Input: part model. Units: mm. Frame: model coordinates. A direction names the side the tool comes from. Coordinates: 2 decimals unless noted, no trailing zeros. Order: outer loops, then holes, each group sorted by start corner. A loop starts at its lowest first (then second) coordinate and runs counter-clockwise, first axis right, second up. Notation, with made-up numbers: (-18, -10) - (20, -10) arc R24 ccw to (20, 17) - close; hole circle Ø5 at (74, 79.25). An arc over 180 degrees is marked (long way). Use a Markdown table: item, result. Add a question column.
from build123d import *

# Parameters (mm, degrees)
BODY_DEPTH                    = 6
SKETCH2_W                     = 10.280011329
SKETCH2_H                     = 42.3
SKETCH2_W_2                   = 2
WINGS_DEPTH                   = 130
SKETCH3_R                     = 1.6
MOUNTING_BORE_DEPTH           = 152.726728034
CUT_EXCESS_MATERIAL_DEPTH     = 175.702604445
CUT_BATTERY_MOUNT_REACH       = 153.727
SKETCH6_R                     = 1.6
SKETCH8_W                     = 6.8
SKETCH8_H                     = 2.8
CAPTURE_NUT_1_DEPTH           = 7.3
CIRPATTERN1_COUNT             = 2
SKETCH10_W                    = 6.8
SKETCH10_H                    = 2.8
CAPTURE_NUT_2_DEPTH           = 7.3
CIRPATTERN2_COUNT             = 2
CUT_CENTER_HOLE_REACH         = 153.727
SKETCH11_R                    = 30
CUT_HARNESS_MOUNT_REACH       = 153.727
SKETCH12_R                    = 2.5
CAPTIVE_NUT_WALL_1_DEPTH      = 2.8
CAPTIVE_NUT_WALL_2_REACH      = 147.131
CAPTIVE_NUT_WALL_3_REACH      = 147.131
CAPTIVE_NUT_WALL_4_REACH      = 147.131
MIDDLE_DECK_HOLES_REACH       = 161.285
SKETCH20_R                    = 1.6
MIDDLE_DECK_CAPTIVE_NUT_DEPTH = 2.5
WING_EXTRA_WIDTH_1_DEPTH      = 3
WING_EXTRA_WIDTH_2_DEPTH      = 3


with BuildPart() as part:
    # Sketch1 → body (new body)
    with BuildSketch(Plane(origin=(0, 0, 0), x_dir=(1, 0, 0), z_dir=(0, 1, 0))):
        with BuildLine():
            ThreePointArc((-39.719988671, -21.15), (-45, 0), (-39.719988671, 21.15))
            Line((-39.719988671, 21.15), (-50, 21.15))
            Line((-50, 21.15), (-50, -21.15))
            Line((-50, -21.15), (-39.719988671, -21.15))
        make_face()
        with BuildLine():
            Line((-16, -21.15), (-16, 21.15))
            Line((-16, 21.15), (-39.719988671, 21.15))
            ThreePointArc((-39.719988671, 21.15), (-45, 0), (-39.719988671, -21.15))
            Line((-39.719988671, -21.15), (-16, -21.15))
        make_face()
        with BuildLine():
            Line((-39.719988671, 21.15), (-16, 21.15))
            Line((-16, 21.15), (-16, -21.15))
            Line((-16, -21.15), (-39.719988671, -21.15))
            ThreePointArc((-39.719988671, -21.15), (0, -45), (39.719988671, -21.15))
            Line((39.719988671, -21.15), (16, -21.15))
            Line((16, -21.15), (16, 21.15))
            Line((16, 21.15), (39.719988671, 21.15))
            ThreePointArc((39.719988671, 21.15), (0, 45), (-39.719988671, 21.15))
        make_face()
        with BuildLine():
            ThreePointArc((45, 0), (43.66004747, 10.899552968), (39.719988671, 21.15))
            Line((39.719988671, 21.15), (16, 21.15))
            Line((16, 21.15), (16, -21.15))
            Line((16, -21.15), (39.719988671, -21.15))
            ThreePointArc((39.719988671, -21.15), (43.66004747, -10.899552968), (45, 0))
        make_face()
        with BuildLine():
            Line((50, 21.15), (39.719988671, 21.15))
            ThreePointArc((39.719988671, 21.15), (43.66004747, 10.899552968), (45, 0))
            ThreePointArc((45, 0), (43.66004747, -10.899552968), (39.719988671, -21.15))
            Line((39.719988671, -21.15), (50, -21.15))
            Line((50, -21.15), (50, 21.15))
        make_face()
    extrude(amount=BODY_DEPTH)

    # Sketch2 → wings (add)
    with BuildSketch(Plane(origin=(0, 6, 0), x_dir=(1, 0, 0), z_dir=(0, 1, 0))):
        with Locations((44.859994336, 0)):
            Rectangle(SKETCH2_W, SKETCH2_H)
        with Locations((-44.859994336, 0)):
            Rectangle(SKETCH2_W, SKETCH2_H)
        with Locations((-38.719988671, 0)):
            Rectangle(SKETCH2_W_2, SKETCH2_H)
        with Locations((38.719988671, 0)):
            Rectangle(SKETCH2_W_2, SKETCH2_H)
    extrude(amount=WINGS_DEPTH)

    # Sketch3 → mounting-bore (cut, through all)
    with BuildSketch(Plane(origin=(0, 136, 0), x_dir=(1, 0, 0), z_dir=(0, 1, 0))):
        with Locations(Location((43, -17.5, 0), (0, 0, 270))):
            Circle(SKETCH3_R)
        with Locations(Location((-43, -17.5, 0), (0, 0, 270))):
            Circle(SKETCH3_R)
        with Locations(Location((-43, 17.5, 0), (0, 0, 270))):
            Circle(SKETCH3_R)
        with Locations(Location((43, 17.5, 0), (0, 0, 270))):
            Circle(SKETCH3_R)
    extrude(amount=-MOUNTING_BORE_DEPTH, mode=Mode.SUBTRACT)

    # Sketch5 → cut-excess-material (cut, through all)
    with BuildSketch(Plane(origin=(50, 0, 0), x_dir=(0, 0, -1), z_dir=(1, 0, 0))):
        Polygon((0, 6), (9, 6), (9, 136), (-9, 136), (-9, 6), align=None)
    extrude(amount=-CUT_EXCESS_MATERIAL_DEPTH, mode=Mode.SUBTRACT)

    # Sketch6 → cut-battery-mount (cut, up to next)
    with BuildSketch(Plane.XZ, mode=Mode.PRIVATE) as cut_battery_mount_sk1:
        with Locations(Location((-44, 0, 0), (0, 0, 270))):
            Circle(SKETCH6_R)
    cut_battery_mount_tool1 = extrude(cut_battery_mount_sk1.sketch, amount=-CUT_BATTERY_MOUNT_REACH, mode=Mode.PRIVATE) & part.part
    # Sketch6 → cut-battery-mount (cut, up to next)
    with BuildSketch(Plane.XZ, mode=Mode.PRIVATE) as cut_battery_mount_sk2:
        with Locations(Location((44, 0, 0), (0, 0, 270))):
            Circle(SKETCH6_R)
    cut_battery_mount_tool2 = extrude(cut_battery_mount_sk2.sketch, amount=-CUT_BATTERY_MOUNT_REACH, mode=Mode.PRIVATE) & part.part
    add(cut_battery_mount_tool1.solids().sort_by_distance((-44, 0, 0))[0], mode=Mode.SUBTRACT)
    add(cut_battery_mount_tool2.solids().sort_by_distance((44, 0, 0))[0], mode=Mode.SUBTRACT)

    # Sketch8 → capture-nut-1 (cut)
    with BuildSketch(Plane.XY.offset(21.15)):
        with Locations((42.999988671, 130)):
            Rectangle(SKETCH8_W, SKETCH8_H)
    capture_nut_1 = extrude(amount=-CAPTURE_NUT_1_DEPTH, mode=Mode.SUBTRACT)

    # CirPattern1: capture-nut-1 ×2 about axis
    cirpattern1_axis = Axis((0, 0, 0), (0, 1, 0))
    for i in range(1, CIRPATTERN1_COUNT):
        add(capture_nut_1.rotate(cirpattern1_axis, i * 360 / CIRPATTERN1_COUNT), mode=Mode.SUBTRACT)

    # Sketch10 → capture-nut-2 (cut)
    with BuildSketch(Plane(origin=(0, 0, -21.15), x_dir=(-1, 0, 0), z_dir=(0, 0, -1))):
        with Locations((-42.999988671, 130)):
            Rectangle(SKETCH10_W, SKETCH10_H)
    capture_nut_2 = extrude(amount=-CAPTURE_NUT_2_DEPTH, mode=Mode.SUBTRACT)

    # CirPattern2: capture-nut-2 ×2 about axis
    cirpattern2_axis = Axis((0, 0, 0), (0, 1, 0))
    for i in range(1, CIRPATTERN2_COUNT):
        add(capture_nut_2.rotate(cirpattern2_axis, i * 360 / CIRPATTERN2_COUNT), mode=Mode.SUBTRACT)

    # Sketch11 → cut-center-hole (cut, up to next)
    with BuildSketch(Plane.XZ, mode=Mode.PRIVATE) as cut_center_hole_sk1:
        with Locations(Location((0, 0, 0), (0, 0, 270))):
            Circle(SKETCH11_R)
    cut_center_hole_tool1 = extrude(cut_center_hole_sk1.sketch, amount=-CUT_CENTER_HOLE_REACH, mode=Mode.PRIVATE) & part.part
    add(cut_center_hole_tool1.solids().sort_by_distance((0, 0, 0))[0], mode=Mode.SUBTRACT)

    # Sketch12 → cut-harness-mount (cut, up to next)
    with BuildSketch(Plane.XZ, mode=Mode.PRIVATE) as cut_harness_mount_sk1:
        with Locations(Location((0, -40, 0), (0, 0, 270))):
            Circle(SKETCH12_R)
    cut_harness_mount_tool1 = extrude(cut_harness_mount_sk1.sketch, amount=-CUT_HARNESS_MOUNT_REACH, mode=Mode.PRIVATE) & part.part
    # Sketch12 → cut-harness-mount (cut, up to next)
    with BuildSketch(Plane.XZ, mode=Mode.PRIVATE) as cut_harness_mount_sk2:
        with Locations(Location((0, 40, 0), (0, 0, 270))):
            Circle(SKETCH12_R)
    cut_harness_mount_tool2 = extrude(cut_harness_mount_sk2.sketch, amount=-CUT_HARNESS_MOUNT_REACH, mode=Mode.PRIVATE) & part.part
    add(cut_harness_mount_tool1.solids().sort_by_distance((0, 0, -40))[0], mode=Mode.SUBTRACT)
    add(cut_harness_mount_tool2.solids().sort_by_distance((0, 0, 40))[0], mode=Mode.SUBTRACT)

    # Sketch13 → captive-nut-wall-1 (add)
    with BuildSketch(Plane(origin=(0, 128.6, 0), x_dir=(1, 0, 0), z_dir=(0, 1, 0))):
        Polygon((46.399988671, 13.85), (46.399988671, 17.5), (44.699994335, 14.555523439), (41.300005665, 14.555523439), (39.600011329, 17.5), (39.599988671, 13.85), align=None)
    extrude(amount=CAPTIVE_NUT_WALL_1_DEPTH)

    # Sketch14 → captive-nut-wall-2 (add, up to next)
    with BuildSketch(Plane(origin=(0, 128.6, 0), x_dir=(1, 0, 0), z_dir=(0, 1, 0)), mode=Mode.PRIVATE) as captive_nut_wall_2_sk1:
        Polygon((-39.599988671, 13.85), (-39.599988671, 17.5), (-41.299994335, 14.555503816), (-44.700005665, 14.555503816), (-46.400011329, 17.5), (-46.400011329, 13.85), align=None)
    captive_nut_wall_2_tool1 = extrude(captive_nut_wall_2_sk1.sketch, amount=CAPTIVE_NUT_WALL_2_REACH, mode=Mode.PRIVATE) - part.part
    add(captive_nut_wall_2_tool1.solids().sort_by_distance((-39.677166, 128.6, -15.675))[0])

    # Sketch16 → captive-nut-wall-3 (add, up to next)
    with BuildSketch(Plane(origin=(0, 128.6, 0), x_dir=(1, 0, 0), z_dir=(0, 1, 0)), mode=Mode.PRIVATE) as captive_nut_wall_3_sk1:
        Polygon((-46.399988671, -13.85), (-46.399988671, -17.5), (-44.699994335, -14.555523439), (-41.300005665, -14.555523439), (-39.600011329, -17.5), (-39.600011329, -13.85), align=None)
    captive_nut_wall_3_tool1 = extrude(captive_nut_wall_3_sk1.sketch, amount=CAPTIVE_NUT_WALL_3_REACH, mode=Mode.PRIVATE) - part.part
    add(captive_nut_wall_3_tool1.solids().sort_by_distance((-46.322812, 128.6, 15.675))[0])

    # Sketch17 → captive-nut-wall-4 (add, up to next)
    with BuildSketch(Plane(origin=(0, 128.6, 0), x_dir=(1, 0, 0), z_dir=(0, 1, 0)), mode=Mode.PRIVATE) as captive_nut_wall_4_sk1:
        Polygon((39.599988671, -13.85), (39.599988671, -17.5), (41.299994335, -14.555503816), (44.700005665, -14.555503816), (46.400011329, -17.5), (46.400011329, -13.85), align=None)
    captive_nut_wall_4_tool1 = extrude(captive_nut_wall_4_sk1.sketch, amount=CAPTIVE_NUT_WALL_4_REACH, mode=Mode.PRIVATE) - part.part
    add(captive_nut_wall_4_tool1.solids().sort_by_distance((39.677166, 128.6, 15.675))[0])

    # Sketch20 → middle-deck-holes (cut, up to next)
    with BuildSketch(Plane.XY.offset(21.15), mode=Mode.PRIVATE) as middle_deck_holes_sk1:
        with Locations((-43.859994335, 86)):
            Circle(SKETCH20_R)
    middle_deck_holes_tool1 = extrude(middle_deck_holes_sk1.sketch, amount=-MIDDLE_DECK_HOLES_REACH, mode=Mode.PRIVATE) & part.part
    # Sketch20 → middle-deck-holes (cut, up to next)
    with BuildSketch(Plane.XY.offset(21.15), mode=Mode.PRIVATE) as middle_deck_holes_sk2:
        with Locations((43.859994335, 86)):
            Circle(SKETCH20_R)
    middle_deck_holes_tool2 = extrude(middle_deck_holes_sk2.sketch, amount=-MIDDLE_DECK_HOLES_REACH, mode=Mode.PRIVATE) & part.part
    add(middle_deck_holes_tool1.solids().sort_by_distance((-43.859994, 86, 21.15))[0], mode=Mode.SUBTRACT)
    add(middle_deck_holes_tool2.solids().sort_by_distance((43.859994, 86, 21.15))[0], mode=Mode.SUBTRACT)

    # Sketch21 → middle-deck-captive-nut (cut)
    with BuildSketch(Plane(origin=(0, 0, 9), x_dir=(-1, 0, 0), z_dir=(0, 0, -1))):
        Polygon((44.609427523, 89.111004644), (41.540501876, 88.204530501), (40.791068688, 85.093525857), (43.110561148, 82.888995356), (46.179486795, 83.795469499), (46.928919982, 86.906474143), align=None)
        Polygon((-43.110561148, 89.111004644), (-46.179486795, 88.204530501), (-46.928919982, 85.093525857), (-44.609427523, 82.888995356), (-41.540501876, 83.795469499), (-40.791068688, 86.906474143), align=None)
    extrude(amount=-MIDDLE_DECK_CAPTIVE_NUT_DEPTH, mode=Mode.SUBTRACT)

    # Sketch22 → wing-extra-width-1 (add)
    with BuildSketch(Plane(origin=(50, 0, 0), x_dir=(0, 0, -1), z_dir=(1, 0, 0))):
        Polygon((21.15, 136), (9, 136), (9, 6), (-9, 6), (-9, 136), (-21.15, 136), (-21.15, 0), (21.15, 0), align=None)
    extrude(amount=WING_EXTRA_WIDTH_1_DEPTH)

    # Sketch24 → wing-extra-width-2 (add)
    with BuildSketch(Plane.ZY.offset(50)):
        Polygon((9, 136), (9, 6), (-9, 6), (-9, 136), (-21.15, 136), (-21.15, 0), (21.15, 0), (21.15, 136), align=None)
    extrude(amount=WING_EXTRA_WIDTH_2_DEPTH)


solid = part.part
1) Cut plane A-A (y = 25.5). Return the cut outline in (x, z), and give its area (3 significant figures).
2) Material intervals for L1, parallel to X at y = 86, z = 15.25; L2, parallel to X at y = 134.45, z = -17.5; L3, parallel to X at y = 100, z = 20.5, sorted ascending.
3) Pull-direction query (Y, two-part tool) for faces 4 (the cylindrical face through (-0.96, 2.96, -42.31)), 5 (the flat face through (42.5, 84.7, 11.5)), 6 (the flat face through (-45, 136, 15)); classes: pulls with the +Y half, pulls with the -Y half, needs draft (parallel to the pull), parting line crosses it, or undercut.
4) Cut plane B-B (x = 0). Return the cut outline in (y, z), and give its area (3 significant figures).
5) Contact query for flat-ended pins moving along their axis: P1, Ø3, axis at x = -20, z = -23.5, coming from the +Y side; P2, Ø0.8, axis at x = -43, y = 130, coming from the -Z side; P3, Ø3, axis at x = 42, y = 129.5, coming from the +Z side; P4, Ø3.5, axis at x = -41.5, z = -17.5, coming from the +Y side. Output: stop coordinate, or through.
6) Reachability of faces 1 (the flat face through (-45, 70, -9)), 2 (the flat face through (-43, 128.6, -19.4)), 3 (the flat face through (-44, 128.6, 19)) from +Z, -Z, +X, -X, +Y, -Y: full face, straight path, thin tool, end or side. Return the list, or none.
Computed:
| question | item | result |
|---|---|---|
| 1 | outline | (-53, -21.15) - (-37.72, -21.15) - (-37.72, -9) - (-53, -9) - close; (-53, 9) - (-37.72, 9) - (-37.72, 21.15) - (-53, 21.15) - close; (37.72, -21.15) - (53, -21.15) - (53, -9) - (37.72, -9) - close; (37.72, 9) - (53, 9) - (53, 21.15) - (37.72, 21.15) - close; hole circle Ø3.2 at (-43, -17.5); hole circle Ø3.2 at (-43, 17.5); hole circle Ø3.2 at (43, -17.5); hole circle Ø3.2 at (43, 17.5) |
| 1 | area | 710 mm2 |
| 2 | L1 | x = -53 to -45.46, -42.26 to -37.72, 37.72 to 42.26, 45.46 to 53 |
| 2 | L2 | x = -53 to -44.6, -41.4 to -37.72, 37.72 to 41.4, 44.6 to 53 |
| 2 | L3 | x = -53 to -37.72, 37.72 to 53 |
| 3 | face 4 | needs draft |
| 3 | face 5 | undercut |
| 3 | face 6 | pulls with the +Y half |
| 4 | outline | (0, -45) - (6, -45) - (6, -42.5) - (0, -42.5) - close; (0, -37.5) - (6, -37.5) - (6, -30) - (0, -30) - close; (0, 30) - (6, 30) - (6, 37.5) - (0, 37.5) - close; (0, 42.5) - (6, 42.5) - (6, 45) - (0, 45) - close |
| 4 | area | 120 mm2 |
| 5 | P1 | stops at y = 6 |
| 5 | P2 | stops at z = -14.56 |
| 5 | P3 | stops at z = 21.15 |
| 5 | P4 | stops at y = 136 |
| 6 | face 1 | +X, -X, +Y |
| 6 | face 2 | -Z |
| 6 | face 3 | +Z |
